Autodesk Inventor part; units mm, degrees
ref_plane "YZ Plane" through (0, 0, 0) normal (1, 0, 0) x (0, 1, 0)
ref_plane "XZ Plane" through (0, 0, 0) normal (0, 1, 0) x (-1, 0, 0)
ref_plane "XY Plane" through (0, 0, 0) normal (0, 0, 1) x (1, 0, 0)
sketch "Sketch1" plane through (0, 0, 0) normal (0, 1, 0) x (-1, 0, 0)
  line L0 (-333.2556, -289.2611) -> (-678.6087, -289.2611) construction
  line L1 (-678.6087, -289.2611) -> (-678.6087, -95) construction
  line L2 (-678.6087, -95) -> (-333.2556, -95) construction
  line L3 (-333.2556, -95) -> (-333.2556, -289.2611) construction
  line L4 (-333.2556, -289.2611) -> (-678.6087, -95) construction
  line L5 (-488.8826, -290.1866) -> (-488.8826, -299.1866) construction
  line L6 (-488.8826, -299.1866) -> (-504.8826, -299.1866) construction
  line L7 (-488.8826, -290.1866) -> (-504.8826, -299.1866) construction
  line L8 (45, -10.5) -> (45, 9.5)
  line L9 (110, 44.5) -> (110, -45.5) construction
  circle A0 centre (110, 44.5) radius 1.5
  line L10 (115, -50.5) -> (115, 50.5) construction
  line L11 (110, -45.5) -> (-40, -45.5) construction
  line L12 (-46, -50.5) -> (115, -50.5) construction
  line L13 (115, 50.5) -> (-46, 50.5) construction
  line L14 (-40, 44.5) -> (110, 44.5) construction
  line L15 (25, -10.5) -> (45, -10.5)
  line L16 (25, 9.5) -> (25, -10.5)
  line L17 (25, -10.5) -> (45, 9.5) construction
  line L18 (45, -10.5) -> (25, 9.5) construction
  line L19 (45, 9.5) -> (25, 9.5)
  line L20 (-46, 50.5) -> (-46, -50.5) construction
  line L21 (-40, -45.5) -> (-40, 44.5) construction
  circle A1 centre (-40, 44.5) radius 1.5
  circle A2 centre (-40, -45.5) radius 1.5
  circle A3 centre (110, -45.5) radius 1.5
  line L22 (110, -45.5) -> (110, -50.5) construction
  line L23 (110, -45.5) -> (115, -45.5) construction
  line L24 (-59, -50.5) -> (-115, -50.5) construction
  line L25 (-115, -50.5) -> (-115, 34.5) construction
  line L26 (-115, 34.5) -> (-59, 34.5) construction
  line L27 (-59, 34.5) -> (-59, -50.5) construction
  line L28 (-62.5, -47) -> (-111.5, -47) construction
  line L29 (-111.5, -47) -> (-111.5, 11) construction
  line L30 (-111.5, 11) -> (-62.5, 11) construction
  line L31 (-62.5, 11) -> (-62.5, -47) construction
  circle A4 centre (-62.5, -47) radius 1.5
  circle A5 centre (-111.5, -47) radius 1.5
  circle A6 centre (-62.5, 11) radius 1.5
  circle A7 centre (-111.5, 11) radius 1.5
  line L32 (-87, -47) -> (-87, -50.5) construction
  line L33 (-125, 75) -> (125, 75)
  line L34 (125, 75) -> (125, -75)
  line L35 (125, -75) -> (-125, -75)
  line L36 (-125, -75) -> (-125, 75)
  line L37 (-125, 75) -> (125, -75) construction
  line L38 (125, 75) -> (-125, -75) construction
  line L39 (0, -57.5) -> (0, -75)
  line L40 (115, 0) -> (125, 0) construction
  circle A8 centre (110, -45.5) radius 3.5
  circle A9 centre (110, 44.5) radius 3.5
  circle A10 centre (-40, 44.5) radius 3.5
  circle A11 centre (-40, -45.5) radius 3.5
  circle A12 centre (-62.5, -47) radius 3.5
  circle A13 centre (-62.5, 11) radius 3.5
  circle A14 centre (-111.5, 11) radius 3.5
  circle A15 centre (-111.5, -47) radius 3.5
  point P0 (0, 0)
  point P1 (35, -0.5)
  dimension "d34" = 396.24
  dimension "d37" = 345.3531
  dimension "d39" = 9
  dimension "d40" = 16
  dimension "d41" = 29.358
  dimension "d42" = 29.358
  dimension "d43" = 194.2611
  dimension "d46" = 161
  dimension "d47" = 101
  dimension "d48" = 3
  dimension "d49" = 150
  dimension "d50" = 90
  dimension "d51" = 5
  dimension "d52" = 20
  dimension "d53" = 20
  dimension "d54" = 50
  dimension "d55" = 80
  dimension "d56" = 56
  dimension "d57" = 85
  dimension "d58" = 49
  dimension "d59" = 58
  dimension "d60" = 3
  dimension "d61" = 3.5
  dimension "d64" = 250
  dimension "d65" = 150
  dimension "d73" = 10
  dimension "d74" = 10
  dimension "d75" = 7
extrude "Extrusion2" add sketch "Sketch1" along normal blind 10 contours L15 L16 L19 L8 | A0 | A1 | A2 | A3 | A4 | A5 | A6 | A7 | L33 L34 L35 L36 | A8 | A9 | A10 | A11 | A12 | A13 | A14 | A15
extrude "Extrusion3" add sketch "Sketch1" along normal blind 2 from surface at 10 contours A8 | A9 | A10 | A11 | A12 | A13 | A14 | A15
properties part number "Main Mount"
Can you work these out from the model? Positions are in its coordinate system, mm. A direction names the side the tool comes from. Coordinates: 2 decimals unless noted, no trailing zeros. Write each loop counter-clockwise with the first axis right and the second up, starting at its lowest first coordinate (ties: lowest second). Pieces come first, ordered by that corner, then holes. Notation, with made-up numbers: (25.5, -28) -> (61.5, -28) arc R11 ccw to (61.5, -12) -> close; hole circle Ø11 at (45, 64.5). An arc over 180 degrees is marked (long way). Answer as CSV lines item,"result".
1) On a 3-axis mill with a long thin cutter (end or side, diameter ignored), from which of +Z, -Z, +X, -X, +Y, -Y can I reach the whole of each face in a straight line? I mean faces 4 (the cylindrical face through (-113.34, 10.99, -46.55)), 5 (the flat face through (38, 12, 45)). Say none if no direction works.
Check result:
face 4,"+Y"
face 5,"+Z, -Z, +X, -X, +Y"
2) Will this pin go through, and if not, where does the flat tip stop? P1, Ø8, axis at x = 75, z = -4.5, coming from the +Y side.
Check result:
P1,"y = 10"
3) If we section it at B-B on z = -31: Please give me the cut outline in (x, y).
Check result:
outline,"(-125, 0) -> (125, 0) -> (125, 10) -> (-125, 10) -> close"
4) If we mould it in two halves opening along Z, with no side actions, what happens to faces 1 (the flat face through (2, 5, 75)), 2 (the cylindrical face through (42.58, 10.986, 42.135)), 3 (the flat face through (112, 12, -49))? For each: +Z half, -Z half, draft (parallel to the pull), parting line (faces both ways), or undercut.
Check result:
face 1,"+Z half"
face 2,"undercut"
face 3,"draft"
5) If I drill on line 1 (Z direction, x = -110, y = 11.15); line 2 (Z direction, x = 62.5, y = 11.4); line 3 (Y direction, x = -50.5, z = 36.5), over which ranges is the centre line in solid material (lowest first)? Write a range as from..to.
Check result:
line 1,"-49..-47, -44..-42, 41..43, 46..48"
line 2,"-50.5..-48.5, -45.5..-43.5, 7.5..9.5, 12.5..14.5"
line 3,"0..10"
6) If we section it at A-A on x = 10.5: Please give me the cut outline in (y, z), then the cut area to 3 significant figures.
Check result:
outline,"(0, -75) -> (10, -75) -> (10, 75) -> (0, 75) -> close"
area,"1,500 mm²"
